Model file for the job. Use its own axes, mm. A direction names the side the tool comes from. Give positions to 0.01 mm unless a question says otherwise; leave off trailing zeros. Loops run counter-clockwise (first coordinate to the right, second up) from the corner with the lowest first, then second, coordinate; pieces in that order, holes last. Notation, with made-up numbers: M 70,40.25 L 117,40.25 A30 cw 117,76.25 Z; hole C 33.5,87 d10. An arc over 180 degrees is marked long. Use CSV: the item, a comma, the result in double quotes. Start each with the question number.
(1) Slice it at A-A on z = 2.5. List the corners of the cut face in (x, y).
(2) Wall check: line 1 along Z through (x, y) = (0.75, -4.5); line 2 along Z through (x, y) = (-1.25, -1.5); line 3 along X through (y, z) = (1, 2). Give the ranges that are in metal, low to high. Write a range as from..to.
(3) Slice it at B-B on x = 5. List the corners of the cut face in (y, z), and give its area (3 significant figures).
(4) Tool access for faces 1 (the face through (4, 2, 4)), 2 (the face through (0, 5, 2)): list every direction of +Z, -Z, +X, -X, +Y, -Y with a clear straight run to the whole face (end or side of a thin tool).
```python
from build123d import *

# Parameters (mm, degrees)
F1_DEPTH = 4
F2_SIZE  = 0.3
F3_R     = 4
F4_DEPTH = 4
F5_R     = 3.99999


# Not quite as in the source:
# - a fillet or chamfer is up to 0.001 mm smaller than in the source, because OpenCascade refuses the exact size


with BuildPart() as f1:
    # F0 (on Top) → F1 (new body)
    with BuildSketch(Plane.XY):
        Polygon((2.8867513459, 5), (-2.8867513459, 5), (-5.7735026919, 0), (-2.8867513459, -5), (2.8867513459, -5), (5.7735026919, 0), align=None)
    extrude(amount=F1_DEPTH)

    # F2
    f2_edges = [f1.edges().sort_by_distance(p)[0] for p in [
        (4.330127, -2.5, 4),
        (0, -5, 4),
        (4.330127, 2.5, 4),
        (-4.330127, -2.5, 4),
        (-4.330127, 2.5, 4),
        (0, 5, 4),
    ]]
    chamfer(f2_edges, length=F2_SIZE)

    # F3 (on face) → F4 (join)
    with BuildSketch(Plane.XY.offset(4)):
        Circle(F3_R)
    extrude(amount=F4_DEPTH)

    # F5 (radius 4 in the source; OpenCascade refuses exactly that, so slightly less here)
    f5_edges = [f1.edges().sort_by_distance(p)[0] for p in [
        (-4, 0, 8),
    ]]
    fillet(f5_edges, radius=F5_R)


solid = f1.part
```
Reply:
1,outline,"M -5.77,0 L -2.89,-5 L 2.89,-5 L 5.77,0 L 2.89,5 L -2.89,5 Z"
2,line 1,"z = 0..4"
2,line 2,"z = 0..7.49"
2,line 3,"x = -5.2..5.2"
3,outline,"M -1.34,0 L 1.34,0 L 1.34,3.7 L 0.74,4 L -0.74,4 L -1.34,3.7 Z"
3,area,"10.5 mm^2"
4,face 1,"+Z"
4,face 2,"+Z, -Z, +X, -X, +Y"
